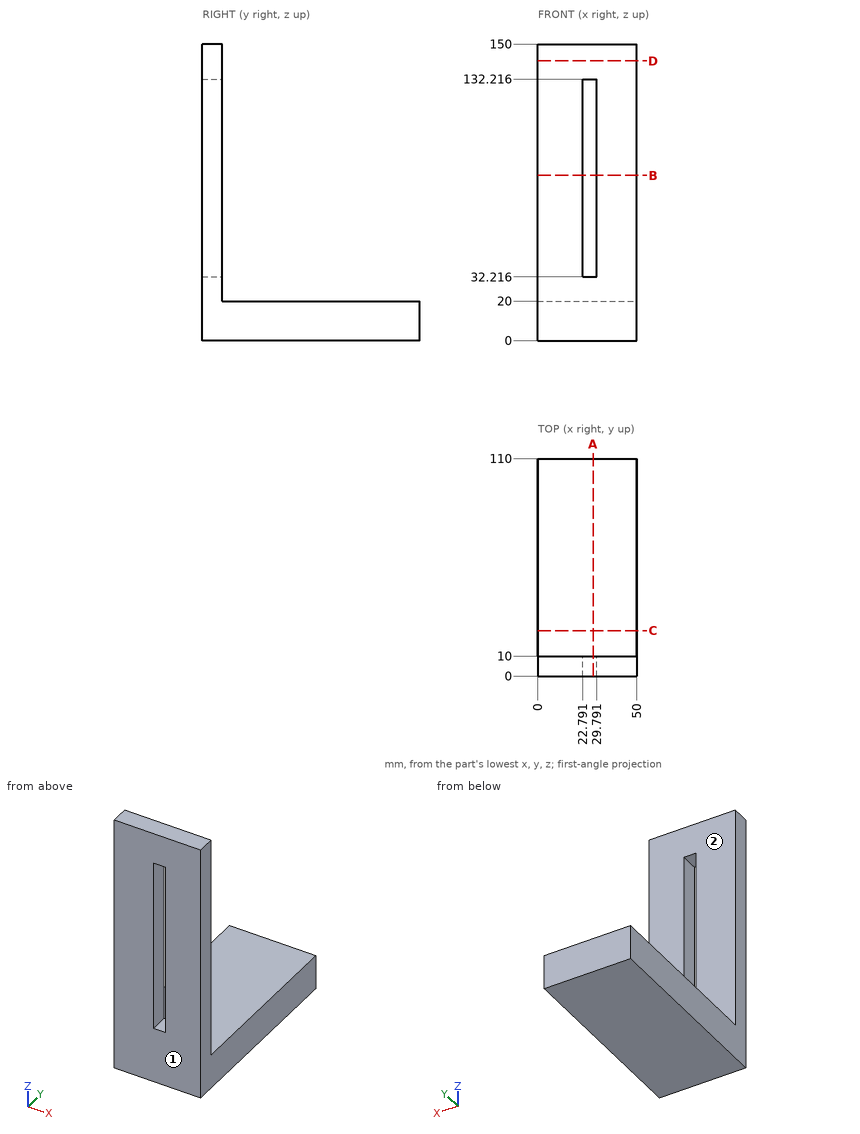
Check sheet for the drawn part. Datum: minimum x, y, z corner. Units: mm. A direction names the side the tool comes from. Give positions to 0.01 mm unless a question says otherwise; leave off trailing zeros. Order: outer loops, then holes, each group sorted by start corner. A loop starts at its lowest first (then second) coordinate and runs counter-clockwise, first axis right, second up.
1. Depth check by flat-ended pin: pin 1 (4 mm diameter, centred on x = 5.5, z = 81.5, fed in from +Y). Enter the tip coordinate at first touch or a pass-through.
Completed:
pin 1: stops at y = 10
2. Access from +Z, -Z, +X, -X, +Y, -Y to the whole of each face (thin tool, end or side, straight path). Record for the marked faces 1 and 2.
Completed:
face 1: +Z, -Z, +X, -X, -Y
face 2: +Z, +X, -X, +Y
3. Sectioned sample at A-A (x = 28). Record the boundary of the cut face in (y, z), then the cut area to 3 significant figures.
Completed:
outline: (0, 0) - (110, 0) - (110, 20) - (10, 20) - (10, 32.22) - (0, 32.22) - close; (0, 132.22) - (10, 132.22) - (10, 150) - (0, 150) - close
area: 2,500 mm2
4. Sectioned sample at D-D (z = 141.5). Record the boundary of the cut face in (x, y), then the cut area to 3 significant figures.
Completed:
outline: (0, 0) - (50, 0) - (50, 10) - (0, 10) - close
area: 500 mm2
5. Sectioned sample at B-B (z = 83.5). Record the boundary of the cut face in (x, y).
Completed:
outline: (0, 0) - (22.79, 0) - (22.79, 10) - (0, 10) - close; (29.79, 0) - (50, 0) - (50, 10) - (29.79, 10) - close
6. Sectioned sample at C-C (y = 23). Record the boundary of the cut face in (x, z).
Completed:
outline: (0, 0) - (50, 0) - (50, 20) - (0, 20) - close
7. Scan lines: line 1 (Z direction, x = 17, y = 62); line 2 (X direction, y = 6.5, z = 59); line 3 (Y direction, x = 15, z = 38). Record each from-to range of solid material in increasing order.
Completed:
line 1: z = 0 to 20
line 2: x = 0 to 22.79, 29.79 to 50
line 3: y = 0 to 10
